Source: three-view drawing plus pictorial views. Frame: mm from the lowest corner of the part. A direction names the side the tool comes from. Round coordinates to 2 decimals unless told otherwise and drop trailing zeros. Order: outer loops, then holes, each group sorted by start corner. A loop starts at its lowest first (then second) coordinate and runs counter-clockwise, first axis right, second up. Notation, with made-up numbers: (67, 13) -> (93, 13) arc R14 ccw to (93, 23) -> close; hole circle Ø7 at (13.5, 42.25). An arc over 180 degrees is marked (long way). Use a Markdown table: item, result.
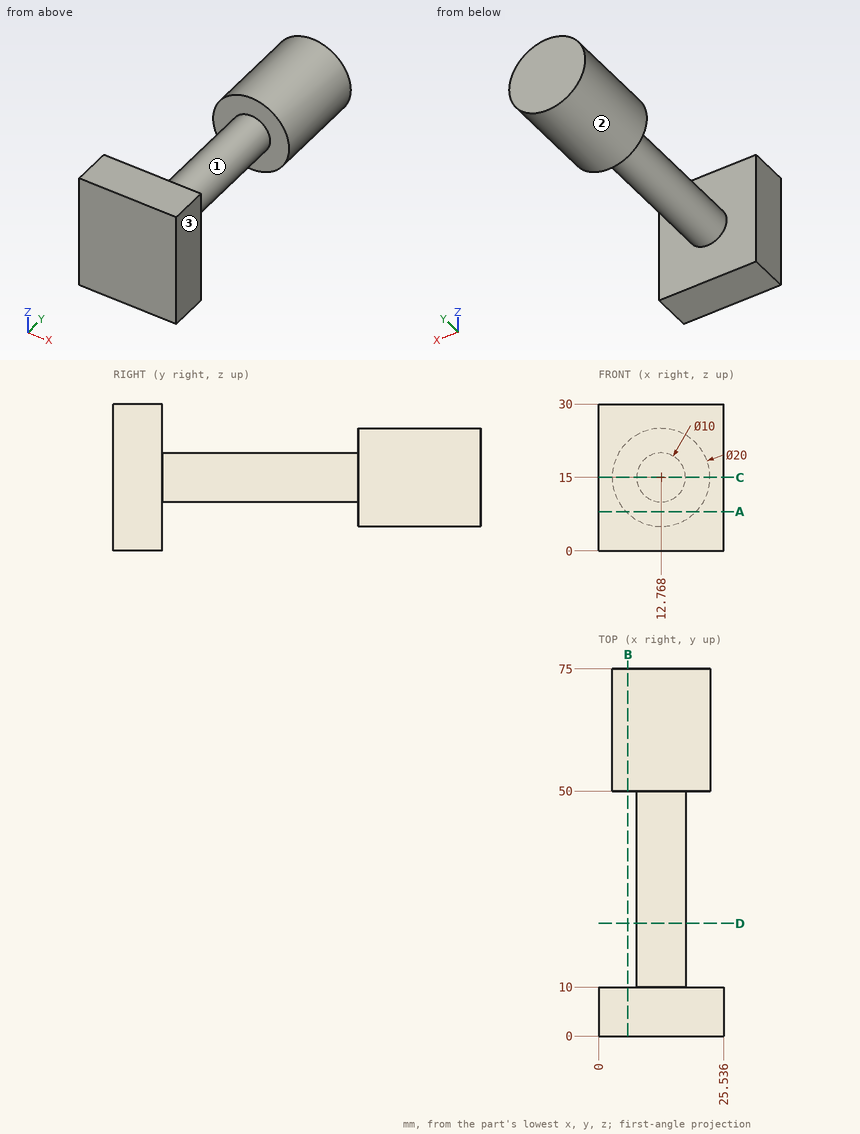
1) Set-up query: the marked faces 1, 2 and 3. Return all of +Z, -Z, +X, -X, +Y, -Y with unobstructed straight access to the full face (end or side cutting, diameter ignored); none if empty.
Results found:
| item | result |
|---|---|
| face 1 | none |
| face 2 | +Y |
| face 3 | +Z, -Z, +X, +Y, -Y |
2) Pin query (flat end, axial travel): pin 1 Ø4 at (y, z) = (62, 25.5) entering from -X; pin 2 Ø1.5 at (x, y) = (21.5, 67.5) entering from +Z; pin 3 Ø5 at (x, z) = (17, 12) entering from -Y; pin 4 Ø1 at (x, y) = (16, 44) entering from -Z. Return the tip coordinate at first contact, or that it passes through.
Results found:
| item | result |
|---|---|
| pin 1 | stops at x = 7.5 |
| pin 2 | stops at z = 21.02 |
| pin 3 | stops at y = 0 |
| pin 4 | stops at z = 10.81 |
3) Cut plane B-B on x = 6. Return loops of the section in (y, z).
Results found:
| item | result |
|---|---|
| outline | (0, 0) -> (10, 0) -> (10, 30) -> (0, 30) -> close; (50, 7.64) -> (75, 7.64) -> (75, 22.36) -> (50, 22.36) -> close |
4) Cut plane D-D on y = 23. Return loops of the section in (x, z).
Results found:
| item | result |
|---|---|
| outline | circle Ø10 at (12.77, 15) |
5) Cut plane A-A on z = 8. Return loops of the section in (x, y), and give its area (3 significant figures).
Results found:
| item | result |
|---|---|
| outline | (0, 0) -> (25.54, 0) -> (25.54, 10) -> (0, 10) -> close; (5.63, 50) -> (19.91, 50) -> (19.91, 75) -> (5.63, 75) -> close |
| area | 612 mm² |
6) Cut plane C-C on z = 15. Return loops of the section in (x, y), and give its area (3 significant figures).
Results found:
| item | result |
|---|---|
| outline | (0, 0) -> (25.54, 0) -> (25.54, 10) -> (17.77, 10) -> (17.77, 50) -> (22.77, 50) -> (22.77, 75) -> (2.77, 75) -> (2.77, 50) -> (7.77, 50) -> (7.77, 10) -> (0, 10) -> close |
| area | 1,160 mm² |
7) Line query: L1, parallel to Y at x = 7.5, z = 12; L2, parallel to Y at x = 23.75, z = 21.75; L3, parallel to Z at x = 13, y = 33 (1 decimal). Output: solid intervals per line, ascending. Write a range as [from, to].
Results found:
| item | result |
|---|---|
| L1 | y = [0, 10], [50, 75] |
| L2 | y = [0, 10] |
| L3 | z = [10, 20] |
